The drawing under review shows one solid part. Ordinate dimensions are in mm from its lowest x, y, z. A direction names the side the tool comes from. Round coordinates to 2 decimals unless told otherwise and drop trailing zeros. Order: outer loops, then holes, each group sorted by start corner. A loop starts at its lowest first (then second) coordinate and runs counter-clockwise, first axis right, second up.
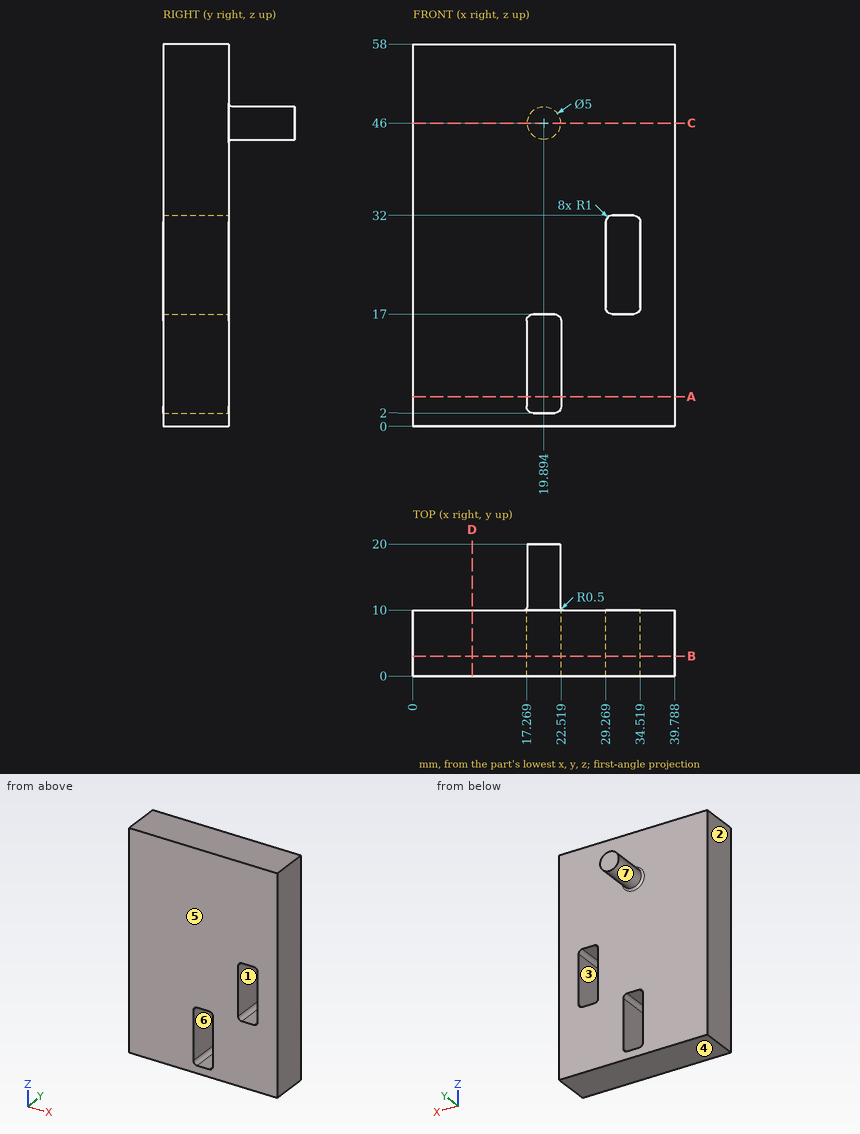
Q1. Mouldability with a two-part tool opening along Z and no side actions: class the marked faces 1, 2, 3 and 4 as +Z half, -Z half, draft (parallel to the pull), parting line (faces both ways), or undercut.
Q2. Wall thickness on line 1 (X direction, y = 9.25, z = 30); line 2 (Y direction, x = 12, z = 47); line 3 (X direction, y = 6.25, z = 17.5) (1 decimal): over which ranges is each line inside the solid? List them lowest first.
Q3. Take a section at A-A, the plane z = 4.5. State the section outline as (x, y) points.
Q4. Tool access review of the marked faces 5, 6 and 7: name each direction out of +Z, -Z, +X, -X, +Y, -Y from which nothing blocks a thin tool from reaching the whole face with its end or side.
Q5. Take a section at B-B, the plane y = 3. State the section outline as (x, z) points, plus the area to 3 significant figures.
Q6. Clearance check with flat-ended pins moving along their axes: pin 1 (4 mm diameter, centred on y = 14, z = 45.5, fed in from +X); pin 2 (12 mm diameter, centred on y = 2.5, z = 15, fed in from -X); pin 3 (5 mm diameter, centred on x = 19, y = 16, fed in from -Z). State where each tip first meets the part, or that it passes through.
Q7. Take a section at D-D, the plane x = 9. State the section outline as (y, z) points, plus the area to 3 significant figures.
Q8. Take a section at C-C, the plane z = 46. State the section outline as (x, y) points.
Working result:
1. face 1: undercut
1. face 2: draft
1. face 3: undercut
1. face 4: -Z half
2. line 1: x = 0 to 29.27, 34.52 to 39.79
2. line 2: y = 0 to 10
2. line 3: x = 0 to 29.4, 34.4 to 39.8
3. outline: (0, 0) - (17.27, 0) - (17.27, 10) - (0, 10) - close; (22.52, 0) - (39.79, 0) - (39.79, 10) - (22.52, 10) - close
4. face 5: +Z, -Z, +X, -X, -Y
4. face 6: +Y, -Y
4. face 7: +Y
5. outline: (0, 0) - (39.79, 0) - (39.79, 58) - (0, 58) - close; hole (17.27, 3) arc R1 ccw to (18.27, 2) - (21.52, 2) arc R1 ccw to (22.52, 3) - (22.52, 16) arc R1 ccw to (21.52, 17) - (18.27, 17) arc R1 ccw to (17.27, 16) - close; hole (29.27, 18) arc R1 ccw to (30.27, 17) - (33.52, 17) arc R1 ccw to (34.52, 18) - (34.52, 31) arc R1 ccw to (33.52, 32) - (30.27, 32) arc R1 ccw to (29.27, 31) - close
5. area: 2,150 mm2
6. pin 1: stops at x = 22.39
6. pin 2: stops at x = 0
6. pin 3: stops at z = 43.5
7. outline: (0, 0) - (10, 0) - (10, 58) - (0, 58) - close
7. area: 580 mm2
8. outline: (0, 0) - (39.79, 0) - (39.79, 10) - (22.89, 10) arc R0.5 cw to (22.39, 10.5) - (22.39, 20) - (17.39, 20) - (17.39, 10.5) arc R0.5 cw to (16.89, 10) - (0, 10) - close
